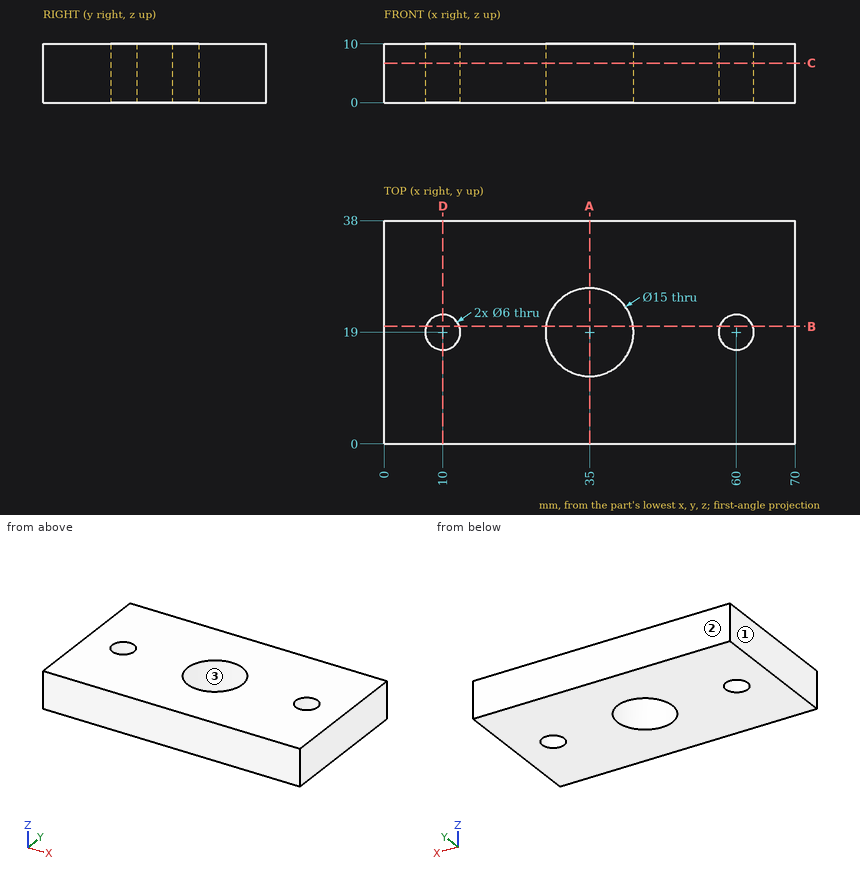
Answer from the drawing. Dimensions are ordinates in mm from the lowest x, y and z of the part. Coordinates: 2 decimals unless noted, no trailing zeros. Write each loop counter-clockwise with the first axis right and the second up, starting at its lowest first coordinate (ties: lowest second). Pieces come first, ordered by that corner, then holes. Notation, with made-up numbers: (0.25, 10) - (31.25, 10) arc R28 cw to (31.25, 32) - close; hole circle Ø7 at (24.25, 26.5). An arc over 180 degrees is marked (long way). Answer as CSV lines item,"result".
1. Given P1, Ø3.5, axis at x = 60, y = 19, coming from the +Z side, flat-ended and moving along its own axis, determine where the tip first touches the part or whether it passes through.
Computed values:
P1,"passes through"
2. Find section A-A (x = 35). Give the vertices of the cut face in (y, z), plus the area to 3 significant figures.
Computed values:
outline,"(0, 0) - (11.5, 0) - (11.5, 10) - (0, 10) - close; (26.5, 0) - (38, 0) - (38, 10) - (26.5, 10) - close"
area,"230 mm²"
3. Determine the mould class of the marked faces 1, 2 and 3 for opening direction X: +X half, -X half, draft (parallel to the pull), parting line (faces both ways), or undercut.
Computed values:
face 1,"-X half"
face 2,"draft"
face 3,"undercut"
4. Find section C-C (z = 6.75). Give the vertices of the cut face in (x, y), plus the area to 3 significant figures.
Computed values:
outline,"(0, 0) - (70, 0) - (70, 38) - (0, 38) - close; hole circle Ø6 at (10, 19); hole circle Ø15 at (35, 19); hole circle Ø6 at (60, 19)"
area,"2,430 mm²"
5. Find section B-B (y = 20). Give the vertices of the cut face in (x, z), plus the area to 3 significant figures.
Computed values:
outline,"(0, 0) - (7.17, 0) - (7.17, 10) - (0, 10) - close; (12.83, 0) - (27.57, 0) - (27.57, 10) - (12.83, 10) - close; (42.43, 0) - (57.17, 0) - (57.17, 10) - (42.43, 10) - close; (62.83, 0) - (70, 0) - (70, 10) - (62.83, 10) - close"
area,"438 mm²"
6. Straight lines are drawn through the part: line 1 (X direction, y = 16.5, z = 6); line 2 (X direction, y = 17, z = 0.75); line 3 (Y direction, x = 35, z = 4.5). For each, find the intervals that lie inside material, in ascending order. Write a range as [from, to].
Computed values:
line 1,"x = [0, 8.34], [11.66, 27.93], [42.07, 58.34], [61.66, 70]"
line 2,"x = [0, 7.76], [12.24, 27.77], [42.23, 57.76], [62.24, 70]"
line 3,"y = [0, 11.5], [26.5, 38]"
7. Find section D-D (x = 10). Give the vertices of the cut face in (y, z).
Computed values:
outline,"(0, 0) - (16, 0) - (16, 10) - (0, 10) - close; (22, 0) - (38, 0) - (38, 10) - (22, 10) - close"
